from build123d import *

# Parameters (mm, degrees)
F0_W     = 228.6
F0_H     = 228.6
F1_DEPTH = 1.5875
F3_D     = 19.84248
F4_D     = 124.587


with BuildPart() as f1:
    # F0 (on Top) → F1 (new body, symmetric)
    with BuildSketch(Plane.XY):
        Rectangle(F0_W, F0_H)
    extrude(amount=F1_DEPTH, both=True)

    # F3 (through all)
    with Locations(Plane.XY.offset(1.5875)):
        with Locations((-76.2, 76.2), (76.2, 76.2), (-76.2, -76.2), (76.2, -76.2)):
            Hole(F3_D / 2)

    # F4 (through all)
    with Locations(Plane.XY.offset(1.5875)):
        with Locations((0, 0)):
            Hole(F4_D / 2)


solid = f1.part
The model under review builds one solid part; all positions refer to its coordinate system, in mm. Give positions to 0.01 mm unless a question says otherwise; leave off trailing zeros. Order: outer loops, then holes, each group sorted by start corner. A loop starts at its lowest first (then second) coordinate and runs counter-clockwise, first axis right, second up. Notation, with made-up numbers: M 73,0.5 L 90,0.5 A14 ccw 90,7.5 Z; hole C -11,-9 d5. An arc over 180 degrees is marked long. Answer in a Markdown table with one row per item. Add a question column.
1. Mouldability with a two-part tool opening along X and no side actions: class faces 1 (the cylindrical face through (67.035, -80, -0.022)), 2 (the flat face through (-52, -49, -1.588)) as released by +X, released by -X, zero draft, split by the parting line, or undercut.
2. Add section B-B on y = -76.2. State the section outline as (x, z) points, plus the area to 3 significant figures.
3. To check wall thickness, follow line 1 along Y through (x, z) = (-76.2, -0.8); line 2 along Y through (x, z) = (-81, -0.6); line 3 along X through (y, z) = (80.5, -0.6). State the ranges of each line that lie inside material, in increasing order.
4. Add section C-C on z = 0.75. State the section outline as (x, y) points, plus the area to 3 significant figures.
5. Add section A-A on y = 0. State the section outline as (x, z) points, plus the area to 3 significant figures.
6. For pin 1 Ø18 at (x, y) = (76.2, 76.2) entering from -Z, flat-tipped, find the tip position at first contact; note if it passes through.
The answers:
| question | item | result |
|---|---|---|
| 1 | face 1 | undercut |
| 1 | face 2 | zero draft |
| 2 | outline | M -114.3,-1.59 L -86.12,-1.59 L -86.12,1.59 L -114.3,1.59 Z; M -66.28,-1.59 L 66.28,-1.59 L 66.28,1.59 L -66.28,1.59 Z; M 86.12,-1.59 L 114.3,-1.59 L 114.3,1.59 L 86.12,1.59 Z |
| 2 | area | 600 mm2 |
| 3 | line 1 | -114.3 to -86.12, -66.28 to 66.28, 86.12 to 114.3 |
| 3 | line 2 | -114.3 to -84.88, -67.52 to 67.52, 84.88 to 114.3 |
| 3 | line 3 | -114.3 to -85.14, -67.26 to 67.26, 85.14 to 114.3 |
| 4 | outline | M -114.3,-114.3 L 114.3,-114.3 L 114.3,114.3 L -114.3,114.3 Z; hole C -76.2,-76.2 d19.84; hole C -76.2,76.2 d19.84; hole C 0,0 d124.59; hole C 76.2,-76.2 d19.84; hole C 76.2,76.2 d19.84 |
| 4 | area | 38,800 mm2 |
| 5 | outline | M -114.3,-1.59 L -62.29,-1.59 L -62.29,1.59 L -114.3,1.59 Z; M 62.29,-1.59 L 114.3,-1.59 L 114.3,1.59 L 62.29,1.59 Z |
| 5 | area | 330 mm2 |
| 6 | pin 1 | through |
